```python
from build123d import *

# Parameters (mm, degrees)
SALIENTE_EXTRUIR1_DEPTH = 20
CROQUIS2_R              = 1.5
CORTAR_EXTRUIR1_DEPTH   = 18.5


with BuildPart() as part:
    # Croquis1 → Saliente-Extruir1 (new body)
    with BuildSketch(Plane(origin=(0, 0, 0), x_dir=(1, 0, 0), z_dir=(0, 1, 0))):
        with BuildLine():
            Line((-19, 0), (-11, 0))
            ThreePointArc((-11, 0), (0, -11), (11, 0))
            Line((11, 0), (19, 0))
            Line((19, 0), (19, -17.5))
            Line((19, -17.5), (-19, -17.5))
            Line((-19, -17.5), (-19, 0))
        make_face()
    extrude(amount=SALIENTE_EXTRUIR1_DEPTH)

    # Croquis2 → Cortar-Extruir1 (cut, through all)
    with BuildSketch(Plane.XY.offset(17.5)):
        with Locations((-15, 16)):
            Circle(CROQUIS2_R)
        with Locations((-15, 4)):
            Circle(CROQUIS2_R)
        with Locations((15, 4)):
            Circle(CROQUIS2_R)
        with Locations((15, 16)):
            Circle(CROQUIS2_R)
    extrude(amount=-CORTAR_EXTRUIR1_DEPTH, mode=Mode.SUBTRACT)


solid = part.part
```
The listing builds one solid part. Answer for the finished solid, in the listing's coordinates (mm). Round coordinates to 2 decimals unless told otherwise and drop trailing zeros. Loops run counter-clockwise (first coordinate to the right, second up) from the corner with the lowest first, then second, coordinate; pieces in that order, holes last.
Q1. Section A-A, the plane y = 4 is taken. Determine the outline of the cut face in (x, z).
Q2. Find the intervals of material crossed by line 1 (Y direction, x = 15, z = 10.5); line 2 (X direction, y = 17, z = 14.5); line 3 (X direction, y = 11, z = 9.25), in increasing order.
Q3. Section C-C, the plane x = 15 is taken. Determine the outline of the cut face in (y, z).
Q4. Section D-D, the plane y = 8.75 is taken. Determine the outline of the cut face in (x, z), then the cut area to 3 significant figures.
Q5. Section B-B, the plane z = 16 is taken. Determine the outline of the cut face in (x, y), then the cut area to 3 significant figures.
Q6. Given pin 1 Ø2.5 at (x, y) = (-15, 4) entering from +Z, flat-ended and moving along its own axis, determine where the tip first touches the part or whether it passes through.
Q7. For a pull along Y with two mould halves and no side action, classify faces 1 (the face through (13.5, 4.07, 8.87)), 2 (the face through (0, 0, 13)), 3 (the face through (0, 10, 11)) as released by +Y, released by -Y, zero draft, split by the parting line, or undercut.
Completed:
1. outline: (-19, 0) - (-16.5, 0) - (-16.5, 17.5) - (-19, 17.5) - close; (-13.5, 0) - (-11, 0) arc R11 cw to (11, 0) - (13.5, 0) - (13.5, 17.5) - (-13.5, 17.5) - close; (16.5, 0) - (19, 0) - (19, 17.5) - (16.5, 17.5) - close
2. line 1: y = 0 to 2.5, 5.5 to 14.5, 17.5 to 20
2. line 2: x = -19 to -16.12, -13.88 to 13.88, 16.12 to 19
2. line 3: x = -19 to -5.95, 5.95 to 19
3. outline: (0, 0) - (2.5, 0) - (2.5, 17.5) - (0, 17.5) - close; (5.5, 0) - (14.5, 0) - (14.5, 17.5) - (5.5, 17.5) - close; (17.5, 0) - (20, 0) - (20, 17.5) - (17.5, 17.5) - close
4. outline: (-19, 0) - (-11, 0) arc R11 cw to (11, 0) - (19, 0) - (19, 17.5) - (-19, 17.5) - close
4. area: 475 mm2
5. outline: (-19, 0) - (19, 0) - (19, 20) - (-19, 20) - close; hole circle Ø3 at (-15, 4); hole circle Ø3 at (-15, 16); hole circle Ø3 at (15, 4); hole circle Ø3 at (15, 16)
5. area: 732 mm2
6. pin 1: passes through
7. face 1: undercut
7. face 2: released by -Y
7. face 3: zero draft
